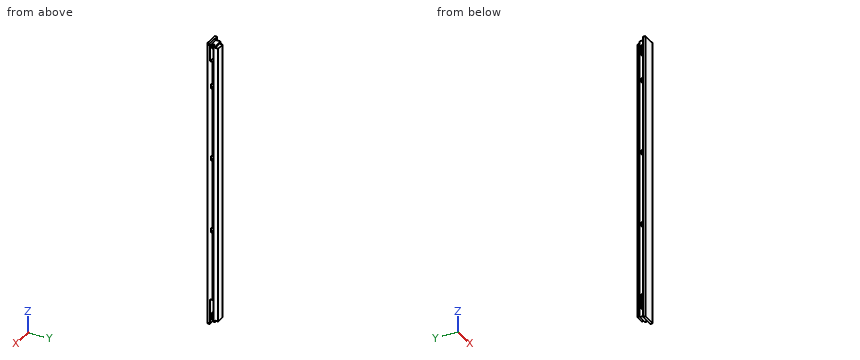
from build123d import *

# Parameters (mm, degrees)
SKETCH003_W     = 90
SKETCH003_H     = 65
PAD001_DEPTH    = 1870
POCKET016_DEPTH = 15
POCKET018_DEPTH = 15
SKETCH006_W     = 10
SKETCH006_H     = 30
POCKET004_DEPTH = 90.001
SKETCH007_W     = 20
SKETCH007_H     = 25
POCKET005_DEPTH = 3836.586112
SKETCH008_W     = 50
SKETCH008_H     = 15
POCKET006_DEPTH = 3836.586112
SKETCH009_W     = 25
SKETCH009_H     = 20
POCKET007_DEPTH = 1870.001
SKETCH010_W     = 15
SKETCH010_H     = 50
POCKET008_DEPTH = 1870.001
SKETCH020_W     = 10
SKETCH020_H     = 32
POCKET017_DEPTH = 1870.001


with BuildPart() as part:
    # Sketch003 (on DatumPlane) → Pad001 (new body)
    with BuildSketch(Plane.XY.offset(935)):
        Rectangle(SKETCH003_W, SKETCH003_H)
    extrude(amount=-PAD001_DEPTH)

    # Sketch019 (on DatumPlane) → Pocket016 (cut)
    with BuildSketch(Plane(origin=(0, 0.5, 0), x_dir=(-1, 0, 0), z_dir=(0, 1, 0))):
        Polygon((-45, 935), (-20, 935), (-20, 890), (45, 890), (45, 820), (-45, 820), align=None)
    extrude(amount=-POCKET016_DEPTH, mode=Mode.SUBTRACT)

    # Sketch021 (on DatumPlane) → Pocket018 (cut)
    with BuildSketch(Plane(origin=(0, 0.5, 0), x_dir=(-1, 0, 0), z_dir=(0, 1, 0))):
        Polygon((45, -770), (-45, -770), (-45, -935), (-20, -935), (-20, -870), (45, -870), align=None)
    extrude(amount=-POCKET018_DEPTH, mode=Mode.SUBTRACT)

    # Sketch006 (on DatumPlane) → Pocket004 (cut, through all)
    with BuildSketch(Plane.YZ.offset(45)):
        with Locations((-4.5, -305)):
            Rectangle(SKETCH006_W, SKETCH006_H)
        with Locations((-4.5, 175)):
            Rectangle(SKETCH006_W, SKETCH006_H)
        with Locations((-4.5, 655)):
            Rectangle(SKETCH006_W, SKETCH006_H)
    extrude(amount=-POCKET004_DEPTH, mode=Mode.SUBTRACT)

    # Sketch007 (on DatumPlane) → Pocket005 (cut, through all)
    with BuildSketch(Plane.YZ.offset(45)):
        with Locations((22.5, 922.5)):
            Rectangle(SKETCH007_W, SKETCH007_H)
    pocket005 = extrude(amount=-POCKET005_DEPTH, mode=Mode.SUBTRACT)

    # Sketch008 (on DatumPlane) → Pocket006 (cut, through all)
    with BuildSketch(Plane.YZ.offset(45)):
        with Locations((7.5, 927.5)):
            Rectangle(SKETCH008_W, SKETCH008_H)
    pocket006 = extrude(amount=-POCKET006_DEPTH, mode=Mode.SUBTRACT)

    # Mirrored002: Pocket005, Pocket006 across XY
    add(pocket005.mirror(Plane.XY), mode=Mode.SUBTRACT)
    add(pocket006.mirror(Plane.XY), mode=Mode.SUBTRACT)

    # Sketch009 (on DatumPlane) → Pocket007 (cut, through all)
    with BuildSketch(Plane.XY.offset(935)):
        with Locations((-32.5, 22.5)):
            Rectangle(SKETCH009_W, SKETCH009_H)
    extrude(amount=-POCKET007_DEPTH, mode=Mode.SUBTRACT)

    # Sketch010 (on Plane of DatumPlane003) → Pocket008 (cut, through all)
    with BuildSketch(Plane.XY.offset(935)):
        with Locations((-37.5, 7.5)):
            Rectangle(SKETCH010_W, SKETCH010_H)
    extrude(amount=-POCKET008_DEPTH, mode=Mode.SUBTRACT)

    # Sketch020 (on DatumPlane) → Pocket017 (cut, through all)
    with BuildSketch(Plane.XY.offset(935)):
        with Locations((40, 16.5)):
            Rectangle(SKETCH020_W, SKETCH020_H)
    extrude(amount=-POCKET017_DEPTH, mode=Mode.SUBTRACT)


solid = part.part
Can you work these out from the model? Positions are in its coordinate system, mm. Give positions to 0.01 mm unless a question says otherwise; leave off trailing zeros. Order: outer loops, then holes, each group sorted by start corner. A loop starts at its lowest first (then second) coordinate and runs counter-clockwise, first axis right, second up. Notation, with made-up numbers: M 72.5,62.25 L 101.5,62.25 A18 ccw 101.5,87.25 Z; hole C 32.25,46 d6. An arc over 180 degrees is marked long. Use a Markdown table: item, result. Add a question column.
Item 1: Will these pins go through, and if not, where does the flat tip stop? pin 1 (5 mm diameter, centred on x = -6, y = -3, fed in from +Z); pin 2 (8 mm diameter, centred on x = 1.5, y = -6, fed in from -Z); pin 3 (9.5 mm diameter, centred on y = 15, z = 393.5, fed in from +X); pin 4 (16.5 mm diameter, centred on x = 16, y = -10.5, fed in from +Z).
Item 2: If I drill on L1, parallel to Z at x = 11, y = -4; L2, parallel to Z at x = 18, y = -13; L3, parallel to Z at x = -10, y = 7.5, over which ranges is the centre line in solid material (lowest first)? Write a range as [from, to].
Item 3: Suppose I cut it at B-B (z = -154.5). List the corners of the cut face in (x, y) for me, then the cut area to 3 significant figures.
Item 4: Suppose I cut it at A-A (x = -2). Count the separate pieces of the cut face and the enclosed holes in it, then the cut area to 3 significant figures.
Answer sheet:
| question | item | result |
|---|---|---|
| 1 | pin 1 | stops at z = 920 |
| 1 | pin 2 | stops at z = -920 |
| 1 | pin 3 | stops at x = 35 |
| 1 | pin 4 | stops at z = 935 |
| 2 | L1 | z = [-920, -870], [-770, -320], [-290, 160], [190, 640], [670, 820], [890, 920] |
| 2 | L2 | z = [-920, -870], [-770, 820], [890, 920] |
| 2 | L3 | z = [-920, 920] |
| 3 | outline | M -45,-32.5 L 45,-32.5 L 45,0.5 L 35,0.5 L 35,32.5 L -20,32.5 L -20,12.5 L -30,12.5 L -30,-17.5 L -45,-17.5 Z |
| 3 | area | 4,580 mm² |
| 4 | separate pieces | 1 |
| 4 | enclosed holes | 5 |
| 4 | area | 116,000 mm² |
